Study the drawing (mm; zero at the part's minimum x, y, z) and answer. Coordinates: 2 decimals unless noted, no trailing zeros. Loops run counter-clockwise (first coordinate to the right, second up) from the corner with the lowest first, then second, coordinate; pieces in that order, holes last. Notation, with made-up numbers: (9, -35.5) - (27, -35.5) arc R19 ccw to (27, -0.5) - close; hole circle Ø9 at (21, 65). An arc over 180 degrees is marked (long way). Use CSV: the item, a comma, the result in double quotes.
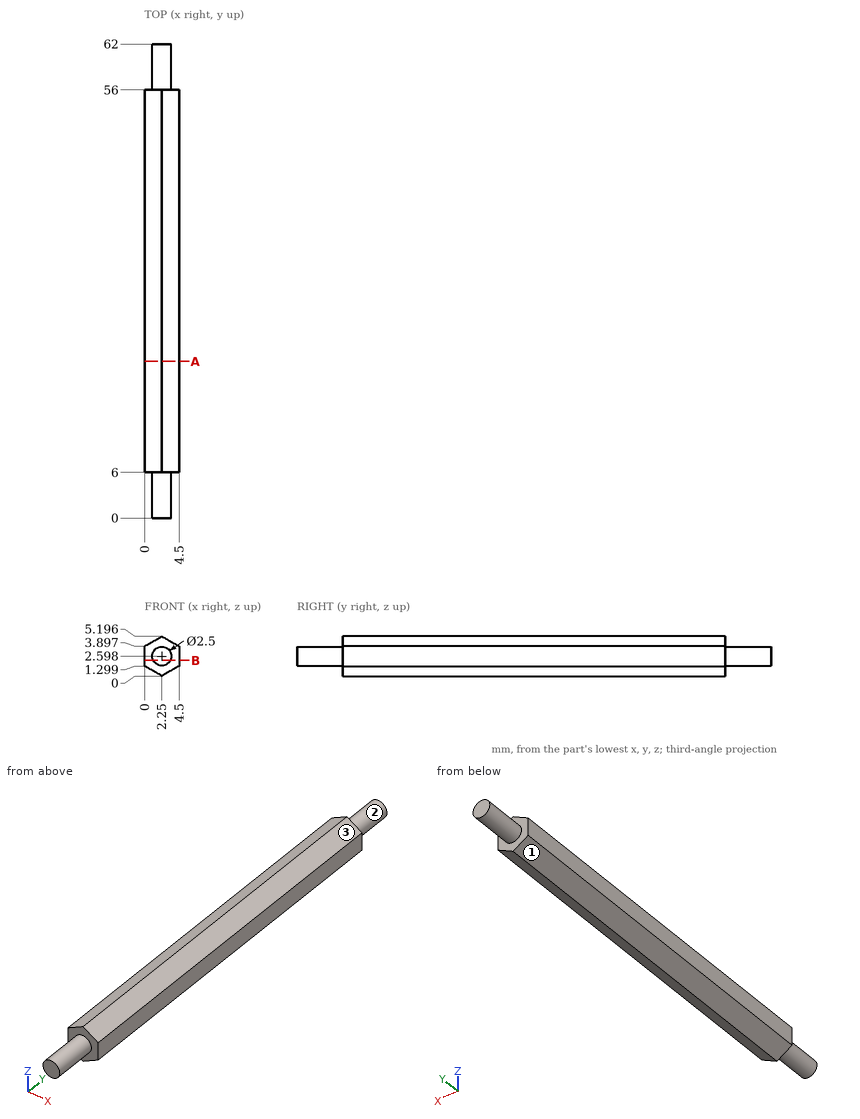
Q1. For a pull along X with two mould halves and no side action, classify the marked faces 1, 2 and 3 as +X half, -X half, draft (parallel to the pull), parting line (faces both ways), or undercut.
Reported:
face 1,"-X half"
face 2,"parting line"
face 3,"+X half"
Q2. Find the intervals of material crossed by probe 1 along Y at (x, z) = (2.75, 1); probe 2 along Z at (x, y) = (2.3, 36.5); probe 3 along X at (y, z) = (14, 4.65) (1 decimal), in increasing order. Write a range as [from, to].
Reported:
probe 1,"y = [6, 56]"
probe 2,"z = [0.03, 5.17]"
probe 3,"x = [1.3, 3.2]"
Q3. The part is cut by section B-B on z = 2.05. Determine the outline of the cut face in (x, y).
Reported:
outline,"(0, 6) - (1.13, 6) - (1.13, 0) - (3.37, 0) - (3.37, 6) - (4.5, 6) - (4.5, 56) - (3.37, 56) - (3.37, 62) - (1.13, 62) - (1.13, 56) - (0, 56) - close"
Q4. The part is cut by section A-A on y = 20.5. Determine the outline of the cut face in (x, z), and give its area (3 significant figures).
Reported:
outline,"(0, 1.3) - (2.25, 0) - (4.5, 1.3) - (4.5, 3.9) - (2.25, 5.2) - (0, 3.9) - close"
area,"17.5 mm²"
